```python
from build123d import *

# Parameters (mm, degrees)
F1_DEPTH  = 18.288
F2_R      = 3.4799850438
F2_R_2    = 2.0474430639
F3_DEPTH  = 1.778
F4_R      = 4.1871679965
F4_R_2    = 1.8588242599
F5_DEPTH  = 19.812
F6_R      = 1.062986484
F6_R_2    = 1.2354744031
F7_DEPTH  = 7.366
F8_W      = 9.1641424224
F8_H      = 0.7049338892
F9_DEPTH  = 1.27
F10_W     = 2.6493370533
F10_H     = 1.4129802585
F11_DEPTH = 17.78
F12_R     = 1.1796889781
F13_DEPTH = 2.794
F14_R     = 1.4881662005
F15_DEPTH = 5.842


with BuildPart() as f1:
    # F0 (on Front) → F1 (new body)
    with BuildSketch(Plane.XZ):
        with BuildLine():
            ThreePointArc((-3.577367444, 3.5675205461), (-1.9301777364, -4.6689586186), (5.0522035466, 0))
            ThreePointArc((5.0522035466, 0), (4.6689586186, 1.9301777364), (3.577367444, 3.5675205461))
            Line((3.577367444, 3.5675205461), (-3.577367444, 3.5675205461))
        make_face()
        with BuildLine():
            Line((-3.577367444, 3.5675205461), (3.577367444, 3.5675205461))
            ThreePointArc((3.577367444, 3.5675205461), (0, 5.0522035466), (-3.577367444, 3.5675205461))
        make_face()
        with BuildLine():
            ThreePointArc((-3.577367444, 3.5675205461), (0, 5.0522035466), (3.577367444, 3.5675205461))
            Line((3.577367444, 3.5675205461), (3.577367444, 8.872252889))
            Line((3.577367444, 8.872252889), (-3.6853936035, 8.872252889))
            Line((-3.6853936035, 8.872252889), (-3.6853936035, 3.5675205461))
            Line((-3.6853936035, 3.5675205461), (-3.577367444, 3.5675205461))
        make_face()
    extrude(amount=F1_DEPTH)

    # F2 (on Front) → F3 (join)
    with BuildSketch(Plane.XZ):
        Circle(F2_R)
        with Locations((0, 6.6883149557)):
            Circle(F2_R_2)
    extrude(amount=-F3_DEPTH)

    # F4 (on Front) → F5 (join)
    with BuildSketch(Plane.XZ):
        Circle(F4_R)
        with Locations((0, 6.961222738)):
            Circle(F4_R_2)
    extrude(amount=F5_DEPTH)

    # F6 (on Top) → F7 (join)
    with BuildSketch(Plane.XY):
        with Locations((0, -14.6069657058)):
            Circle(F6_R)
        with Locations((0, -5.7952911593)):
            Circle(F6_R_2)
    extrude(amount=-F7_DEPTH)

    # F8 (on Right) → F9 (join)
    with BuildSketch(Plane.YZ):
        with Locations((-9.7809578292, -6.4325220883)):
            Rectangle(F8_W, F8_H)
    extrude(amount=F9_DEPTH)

    # F10 (on Front) → F11 (join)
    with BuildSketch(Plane.XZ):
        with Locations((0, 3.6207614467)):
            Rectangle(F10_W, F10_H)
    extrude(amount=-F11_DEPTH)

    # F12 (on Right) → F13 (join)
    with BuildSketch(Plane.YZ):
        Polygon((11.320493184, 5.5902907625), (5.8451956138, 5.5902907625), (6.0218176804, 1.7045951681), (11.320493184, 1.7045951681), align=None)
        Polygon((11.320493184, 1.7045951681), (6.0218176804, 1.7045951681), (6.0218176804, -2.8875903226), (9.5542669296, -2.7109677903), align=None)
        with Locations((8.6711554322, 0)):
            Circle(F12_R, mode=Mode.SUBTRACT)
    extrude(amount=F13_DEPTH)

    # F14 (on Front) → F15 (join)
    with BuildSketch(Plane.XZ):
        Circle(F14_R)
    extrude(amount=-F15_DEPTH)


solid = f1.part
```
Input: part model. Units: mm. Frame: model coordinates. A direction names the side the tool comes from. Give positions to 0.01 mm unless a question says otherwise; leave off trailing zeros. Write each loop counter-clockwise with the first axis right and the second up, starting at its lowest first coordinate (ties: lowest second). Pieces come first, ordered by that corner, then holes. Notation, with made-up numbers: (59, 68) - (81, 68) arc R20 ccw to (81, 107) - close; hole circle Ø10 at (56, 25). An arc over 180 degrees is marked (long way). Write item = value, one per line. Start each with the question number.
1) Reachability of faces 1 (the face through (1, -19.04, 8.53)), 2 (the face through (-0.323, 3.782, -1.453)), 3 (the face through (0, 9, 5)), 4 (the face through (-0.3, 8.8, 4.327)), 5 (the face through (1.688, 5.932, 3.675)) from +Z, -Z, +X, -X, +Y, -Y: full face, straight path, thin tool, end or side. Return the list, or none.
2) Material intervals for L1, parallel to Y at x = -3, z = 4.5; L2, parallel to Y at x = 3, z = -0.75; L3, parallel to Z at x = 1.25, y = 12, sorted ascending. Write a range as [from, to].
3) Pin query (flat end, axial travel): pin 1 (6 mm diameter, centred on y = -4.5, z = 6.5, fed in from +X); pin 2 (4 mm diameter, centred on x = -3.5, z = 2, fed in from +Y); pin 3 (2 mm diameter, centred on x = -1.5, y = -13, fed in from -Z). Return the tip coordinate at first contact, or that it passes through.
4) Cut plane A-A (y = -11). Return loops of the section in (x, z), and give its area (3 significant figures).
5) Draft query along Z for faces 6 (the face through (0, -19.812, 0)), 7 (the face through (1, 9, 5.59)), 8 (the face through (1, -10, -6.08)). Return one class per face: pulls with the +Z half, pulls with the -Z half, needs draft (parallel to the pull), parting line crosses it, or undercut.
6) Cut plane B-B (y = 15.5). Return loops of the section in (x, z).
Answers follow:
q1.face_1 = -Y
q1.face_2 = none
q1.face_3 = +Z, -X, +Y
q1.face_4 = -X
q1.face_5 = +X
q2.L1 = [-18.29, 0]
q2.L2 = [-19.81, 1.78]
q2.L3 = [2.91, 4.33]
q3.pin_1 = 3.64
q3.pin_2 = 1.78
q3.pin_3 = -5.03
q4.outline = (-3.69, 3.57) - (-3.58, 3.57) arc R5.05 ccw (long way) to (3.58, 3.57) - (3.58, 8.87) - (-3.69, 8.87) - close; (0, -6.78) - (1.27, -6.78) - (1.27, -6.08) - (0, -6.08) - close
q4.area = 112 mm^2
q5.face_6 = needs draft
q5.face_7 = pulls with the +Z half
q5.face_8 = undercut
q6.outline = (-1.32, 2.91) - (1.32, 2.91) - (1.32, 4.33) - (-1.32, 4.33) - close
